Can you work these out from the model? Positions are in its coordinate system, mm. Give positions to 0.01 mm unless a question says otherwise; leave off trailing zeros. Order: outer loops, then holes, each group sorted by start corner. A loop starts at its lowest first (then second) coordinate and runs counter-clockwise, first axis right, second up.
Item 1: I want a section at C-C, the plane y = 0.65. Write out the boundary of the cut face in (x, z).
Item 2: I want a section at A-A, the plane x = 11. Write out the boundary of the cut face in (y, z), then the cut area to 3 significant figures.
Item 3: I want a section at B-B, the plane z = 7. Write out the boundary of the cut face in (x, y), then the cut area to 3 significant figures.
Item 4: If I drill on line 1 along X through (y, z) = (0.35, -2.5); line 2 along Z through (x, y) = (-6, 0.6); line 3 along X through (y, z) = (0.3, 13), over which ranges is the centre line in solid material (lowest first)?
Autodesk Fusion 360 part; units mm, degrees
sketch "Sketch1" plane through (0, 0, 0) normal (0, 1, 0) x (1, 0, 0)
  line L0 (22.5, 17.5) -> (-22.5, 17.5)
  line L1 (-22.5, 17.5) -> (-22.5, -17.5)
  line L2 (-22.5, -17.5) -> (22.5, -17.5)
  line L3 (22.5, -17.5) -> (22.5, 17.5)
  line L4 (22.5, 17.5) -> (-22.5, -17.5) construction
  line L5 (-22.5, 17.5) -> (22.5, -17.5) construction
  line L6 (21, -12.9623) -> (-21, -12.9623)
  line L7 (-21, -12.9623) -> (-21, -15.4623)
  line L8 (-21, -15.4623) -> (21, -15.4623)
  line L9 (21, -15.4623) -> (21, -12.9623)
  line L10 (21, -12.9623) -> (-21, -15.4623) construction
  line L11 (-21, -12.9623) -> (21, -15.4623) construction
  line L12 (19.42, 15.1045) -> (-19.42, 15.1045)
  line L13 (-19.42, 15.1045) -> (-19.42, -15.1045)
  line L14 (-19.42, -15.1045) -> (19.42, -15.1045)
  line L15 (19.42, -15.1045) -> (19.42, 15.1045)
  line L16 (19.42, 15.1045) -> (-19.42, -15.1045) construction
  line L17 (-19.42, 15.1045) -> (19.42, -15.1045) construction
  point P0 (0, -14.2123)
  dimension "d1" = 45
  dimension "d2" = 35
  dimension "d3" = 42
  dimension "d4" = 2.5
extrude "Extrude1" add sketch "Sketch1" along normal blind 3
fillet "Fillet1" radius 2 4 edges at (22.5, 1.5, 17.5) (22.5, 1.5, -17.5) (-22.5, 1.5, 17.5) (-22.5, 1.5, -17.5)
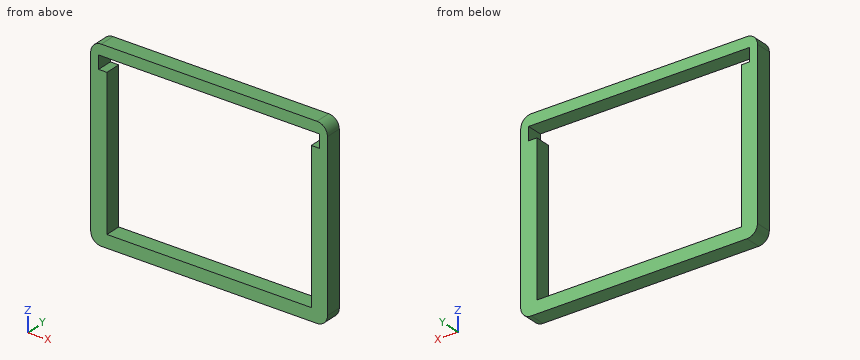
Results list:
1. outline: (-22.5, -15.5) arc R2 ccw to (-20.5, -17.5) - (20.5, -17.5) arc R2 ccw to (22.5, -15.5) - (22.5, 15.5) arc R2 ccw to (20.5, 17.5) - (-20.5, 17.5) arc R2 ccw to (-22.5, 15.5) - close; hole (-21, 12.96) - (-19.42, 12.96) - (-19.42, -15.1) - (19.42, -15.1) - (19.42, 12.96) - (21, 12.96) - (21, 15.46) - (-21, 15.46) - close
2. outline: (0, -17.5) - (3, -17.5) - (3, -15.1) - (0, -15.1) - close; (0, 15.46) - (3, 15.46) - (3, 17.5) - (0, 17.5) - close
2. area: 13.3 mm2
3. outline: (-22.5, 0) - (-19.42, 0) - (-19.42, 3) - (-22.5, 3) - close; (19.42, 0) - (22.5, 0) - (22.5, 3) - (19.42, 3) - close
3. area: 18.5 mm2
4. line 1: x = -22.5 to -19.42, 19.42 to 22.5
4. line 2: z = -17.5 to -15.1, 15.46 to 17.5
4. line 3: x = -22.5 to -21, 21 to 22.5
